from build123d import *

# Parameters (mm, degrees)
SKETCH1_R               = 47.5
SKETCH1_R_2             = 46
BOSS_EXTRUDE1_DEPTH     = 250
SKETCH2_R               = 1
CUT_EXTRUDE1_DEPTH      = 250
CUT_EXTRUDE1_DEPTH_BACK = 250
SKETCH3_W               = 95
SKETCH3_H               = 20
CUT_EXTRUDE2_DEPTH      = 75
CUT_EXTRUDE2_DEPTH_BACK = 79
SKETCH4_R               = 9.5
CUT_EXTRUDE3_DEPTH      = 64
CUT_EXTRUDE3_DEPTH_BACK = 73
BOSS_EXTRUDE2_REACH     = 8
SKETCH5_R               = 12.5
SKETCH5_R_2             = 9.5
SKETCH10_R              = 12.5
SKETCH10_R_2            = 4
BOSS_EXTRUDE7_DEPTH     = 3
BOSS_EXTRUDE8_REACH     = 8
SKETCH12_R              = 12.5
SKETCH12_R_2            = 9.5
SKETCH13_R              = 12.5
SKETCH13_R_2            = 4
BOSS_EXTRUDE9_DEPTH     = 3
BOSS_EXTRUDE11_DEPTH    = 58
SKETCH18_R              = 2
SKETCH18_R_2            = 20
CUT_EXTRUDE5_DEPTH      = 58
CUT_EXTRUDE6_DEPTH      = 98
CUT_EXTRUDE6_DEPTH_BACK = 82


with BuildPart() as part:
    # Sketch1 → Boss-Extrude1 (new body)
    with BuildSketch(Plane.XY):
        Circle(SKETCH1_R)
        Circle(SKETCH1_R_2, mode=Mode.SUBTRACT)
    extrude(amount=BOSS_EXTRUDE1_DEPTH)

    # Sketch2 → Cut-Extrude1 (cut, two sides)
    with BuildSketch(Plane(origin=(0, 0, 0), x_dir=(1, 0, 0), z_dir=(0, 1, 0))) as cut_extrude1_sk:
        with Locations((0, -120)):
            Circle(SKETCH2_R)
    extrude(amount=CUT_EXTRUDE1_DEPTH, mode=Mode.SUBTRACT)
    extrude(cut_extrude1_sk.sketch, amount=-CUT_EXTRUDE1_DEPTH_BACK, mode=Mode.SUBTRACT)

    # Sketch3 → Cut-Extrude2 (cut, two sides)
    with BuildSketch(Plane(origin=(0, 0, 0), x_dir=(1, 0, 0), z_dir=(0, 1, 0))) as cut_extrude2_sk:
        with Locations((0, -10)):
            Rectangle(SKETCH3_W, SKETCH3_H)
    extrude(amount=CUT_EXTRUDE2_DEPTH, mode=Mode.SUBTRACT)
    extrude(cut_extrude2_sk.sketch, amount=-CUT_EXTRUDE2_DEPTH_BACK, mode=Mode.SUBTRACT)

    # Sketch4 → Cut-Extrude3 (cut, two sides)
    with BuildSketch(Plane(origin=(0, 0, 0), x_dir=(1, 0, 0), z_dir=(0, 1, 0))) as cut_extrude3_sk:
        with Locations((0, -220)):
            Circle(SKETCH4_R)
    extrude(amount=CUT_EXTRUDE3_DEPTH, mode=Mode.SUBTRACT)
    extrude(cut_extrude3_sk.sketch, amount=-CUT_EXTRUDE3_DEPTH_BACK, mode=Mode.SUBTRACT)

    # Sketch5 → Boss-Extrude2 (add, up to next)
    with BuildSketch(Plane(origin=(0, 41.5, 0), x_dir=(1, 0, 0), z_dir=(0, 1, 0)), mode=Mode.PRIVATE) as boss_extrude2_sk1:
        with Locations((0, -220)):
            Circle(SKETCH5_R)
        with Locations((0, -220)):
            Circle(SKETCH5_R_2, mode=Mode.SUBTRACT)
    boss_extrude2_tool1 = extrude(boss_extrude2_sk1.sketch, amount=BOSS_EXTRUDE2_REACH, mode=Mode.PRIVATE) - part.part
    add(boss_extrude2_tool1.solids().sort_by_distance((-12.146447, 41.5, 220))[0])

    # Sketch10 → Boss-Extrude7 (add)
    with BuildSketch(Plane.XZ.offset(-41.5)):
        with Locations((0, 220)):
            Circle(SKETCH10_R)
        with Locations((0, 220)):
            Circle(SKETCH10_R_2, mode=Mode.SUBTRACT)
    extrude(amount=BOSS_EXTRUDE7_DEPTH)

    # Sketch12 → Boss-Extrude8 (add, up to next)
    with BuildSketch(Plane(origin=(0, -41.5, 0), x_dir=(1, 0, 0), z_dir=(0, 1, 0)), mode=Mode.PRIVATE) as boss_extrude8_sk1:
        with Locations((0, -220)):
            Circle(SKETCH12_R)
        with Locations((0, -220)):
            Circle(SKETCH12_R_2, mode=Mode.SUBTRACT)
    boss_extrude8_tool1 = extrude(boss_extrude8_sk1.sketch, amount=-BOSS_EXTRUDE8_REACH, mode=Mode.PRIVATE) - part.part
    add(boss_extrude8_tool1.solids().sort_by_distance((-12.146447, -41.5, 220))[0])

    # Sketch13 → Boss-Extrude9 (add)
    with BuildSketch(Plane(origin=(0, -41.5, 0), x_dir=(1, 0, 0), z_dir=(0, 1, 0))):
        with Locations((0, -220)):
            Circle(SKETCH13_R)
        with Locations((0, -220)):
            Circle(SKETCH13_R_2, mode=Mode.SUBTRACT)
    extrude(amount=BOSS_EXTRUDE9_DEPTH)

    # Sketch17 → Boss-Extrude11 (add)
    with BuildSketch(Plane.XY.offset(20)):
        with BuildLine():
            Line((0, 47.5), (-106.5, 47.5))
            Line((-106.5, 47.5), (-106.5, 44.5))
            Line((-106.5, 44.5), (-16.613247726, 44.5))
            ThreePointArc((-16.613247726, 44.5), (-8.440971508, 46.74398357), (0, 47.5))
        make_face()
    extrude(amount=BOSS_EXTRUDE11_DEPTH)

    # Sketch18 → Cut-Extrude5 (cut)
    with BuildSketch(Plane(origin=(0, 47.5, 0), x_dir=(1, 0, 0), z_dir=(0, 1, 0))):
        with Locations((-101, -72.5)):
            Circle(SKETCH18_R)
        with Locations((-101, -25.5)):
            Circle(SKETCH18_R)
        with Locations((-54, -25.5)):
            Circle(SKETCH18_R)
        with Locations((-54, -72.5)):
            Circle(SKETCH18_R)
        with Locations((-77.5, -49)):
            Circle(SKETCH18_R_2)
    extrude(amount=-CUT_EXTRUDE5_DEPTH, mode=Mode.SUBTRACT)

    # Sketch19 → Cut-Extrude6 (cut, two sides)
    with BuildSketch(Plane(origin=(0, 0, 0), x_dir=(0, 0, -1), z_dir=(1, 0, 0))) as cut_extrude6_sk:
        Polygon((-180, 0), (-180, -2), (-250, -2), (-250, 0), (-250, 2), (-180, 2), align=None)
    extrude(amount=CUT_EXTRUDE6_DEPTH, mode=Mode.SUBTRACT)
    extrude(cut_extrude6_sk.sketch, amount=-CUT_EXTRUDE6_DEPTH_BACK, mode=Mode.SUBTRACT)


solid = part.part
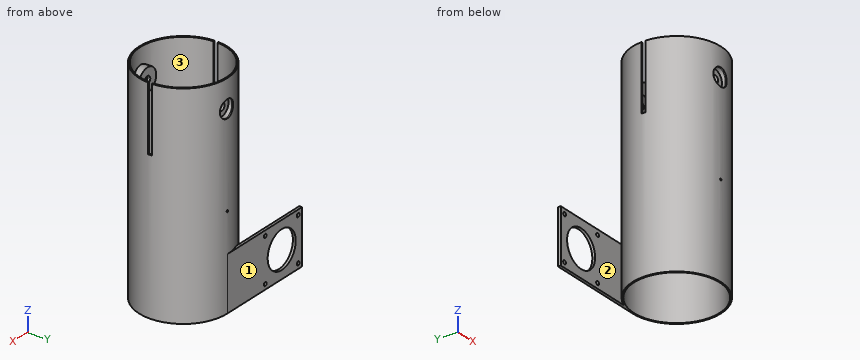
Geometry: final body of the model. Coordinates: model frame, mm. Face numbers are marked on the shaded views. Round coordinates to 2 decimals unless told otherwise and drop trailing zeros. Order: outer loops, then holes, each group sorted by start corner. A loop starts at its lowest first (then second) coordinate and runs counter-clockwise, first axis right, second up.
Q1. Material intervals for probe 1 along Z at (x, y) = (-54, 46); probe 2 along Y at (x, z) = (0, 137), sorted ascending.
Result sheet:
probe 1: z = 20 to 23.5, 27.5 to 70.5, 74.5 to 78
probe 2: y = -47.5 to -46, 46 to 47.5
Q2. Mould query, pull axis Y, two halves, no side actions, for the marked faces 1, 2 and 3. Classes: released by +Y, released by -Y, zero draft, split by the parting line, or undercut.
Result sheet:
face 1: released by +Y
face 2: undercut
face 3: undercut
Q3. Section A-A, the plane x = -77.5. Output: boundary loops of the cut face in (y, z), and give its area (3 significant figures).
Result sheet:
outline: (44.5, 20) - (47.5, 20) - (47.5, 29) - (44.5, 29) - close; (44.5, 69) - (47.5, 69) - (47.5, 78) - (44.5, 78) - close
area: 54.0 mm2
Q4. Section B-B, the plane z = 186.5. Output: boundary loops of the cut face in (x, y).
Result sheet:
outline: (-47.46, -2) arc R47.5 ccw to (47.46, -2) - (45.96, -2) arc R46 cw to (-45.96, -2) - close; (-47.46, 2) - (-45.96, 2) arc R46 cw to (45.96, 2) - (47.46, 2) arc R47.5 ccw to start
Q5. Section D-D, the plane x = -26. Output: boundary loops of the cut face in (y, z).
Result sheet:
outline: (-39.75, 20) - (-37.95, 20) - (-37.95, 250) - (-39.75, 250) - close; (37.95, 20) - (39.75, 20) - (39.75, 250) - (37.95, 250) - close; (44.5, 20) - (47.5, 20) - (47.5, 78) - (44.5, 78) - close
Q6. Pin query (flat end, axial travel): pin 1 (20 mm diameter, centred on x = -1, z = 225.5, fed in from -Y); pin 2 (8 mm diameter, centred on x = -28.5, z = 151.5, fed in from -Y); pin 3 (8 mm diameter, centred on y = 4.5, z = 46.5, fed in from +X); pin 4 (0.8 mm diameter, centred on x = -47, y = 0, fed in from +Z). Return the tip coordinate at first contact, or that it passes through.
Result sheet:
pin 1: stops at y = -47.5
pin 2: stops at y = -40.69
pin 3: stops at x = 47.5
pin 4: stops at z = 180
Q7. Section C-C, the plane z = 49. Output: boundary loops of the cut face in (x, y).
Result sheet:
outline: (-106.5, 44.5) - (-97.5, 44.5) - (-97.5, 47.5) - (-106.5, 47.5) - close; (-57.5, 44.5) - (-16.61, 44.5) arc R47.5 ccw (long way) to (0, 47.5) - (-57.5, 47.5) - close; hole circle Ø92 at (0, 0)
